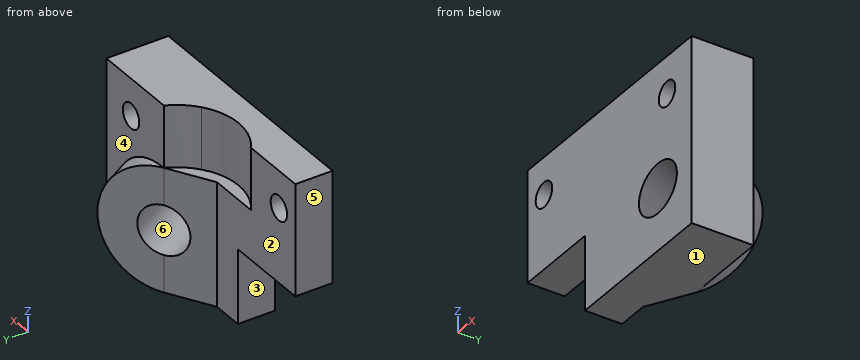
```python
from build123d import *

# Parameters (mm, degrees)
IZIM1_W                     = 35
IZIM1_H                     = 75
Y_KSEKLIK_EKSTR_ZYON1_DEPTH = 25
Y_KSEKLIK_EKSTR_ZYON2_DEPTH = 15
KES_EKSTR_ZYON1_DEPTH       = 25
Y_KSEKLIK_EKSTR_ZYON3_DEPTH = 25
IZIM3_R                     = 5
KES_EKSTR_ZYON2_DEPTH       = 25
IZIM4_R                     = 5
KES_EKSTR_ZYON3_DEPTH       = 26
Y_KSEKLIK_EKSTR_ZYON4_DEPTH = 50
Y_KSEKLIK_EKSTR_ZYON5_REACH = 41.151
IZIM7_R                     = 10
KES_EKSTR_ZYON4_DEPTH       = 40.150635095


with BuildPart() as part:
    # izim1 → Y_kseklik-Ekstr_zyon1 (new body)
    with BuildSketch(Plane(origin=(0, 0, 0), x_dir=(1, 0, 0), z_dir=(0, 1, 0))):
        with Locations((-17.5, 37.5)):
            Rectangle(IZIM1_W, IZIM1_H)
    extrude(amount=Y_KSEKLIK_EKSTR_ZYON1_DEPTH)

    # izim1_4 → Y_kseklik-Ekstr_zyon2 (add)
    with BuildSketch(Plane(origin=(0, 0, 0), x_dir=(1, 0, 0), z_dir=(0, 1, 0))):
        Polygon((-35, 75), (-65, 75), (-65, 45), (-100, 45), (-100, 0), (-35, 0), align=None)
    extrude(amount=Y_KSEKLIK_EKSTR_ZYON2_DEPTH)

    # izim2 → Kes-Ekstr_zyon1 (cut)
    with BuildSketch(Plane.XY):
        with BuildLine():
            Line((-42.912878475, 15), (-72.912878475, 15))
            ThreePointArc((-72.912878475, 15), (-57.912878475, 10), (-42.912878475, 15))
        make_face()
    extrude(amount=-KES_EKSTR_ZYON1_DEPTH, mode=Mode.SUBTRACT)

    # izim2_3 → Y_kseklik-Ekstr_zyon3 (add)
    with BuildSketch(Plane.XY):
        with BuildLine():
            ThreePointArc((-35, 25), (-38.30811914, 19.486992186), (-42.912878475, 15))
            Line((-42.912878475, 15), (-35, 15))
            Line((-35, 15), (-35, 25))
        make_face()
    extrude(amount=-Y_KSEKLIK_EKSTR_ZYON3_DEPTH)

    # izim3 → Kes-Ekstr_zyon2 (cut)
    with BuildSketch(Plane(origin=(0, 15, 0), x_dir=(1, 0, 0), z_dir=(0, 1, 0))):
        with Locations((-90, 15)):
            Circle(IZIM3_R)
    extrude(amount=-KES_EKSTR_ZYON2_DEPTH, mode=Mode.SUBTRACT)

    # izim4 → Kes-Ekstr_zyon3 (cut, through all)
    with BuildSketch(Plane(origin=(0, 25, 0), x_dir=(1, 0, 0), z_dir=(0, 1, 0))):
        with Locations((-15, 15)):
            Circle(IZIM4_R)
    extrude(amount=-KES_EKSTR_ZYON3_DEPTH, mode=Mode.SUBTRACT)

    # izim5 → Y_kseklik-Ekstr_zyon4 (add)
    with BuildSketch(Plane.XY.offset(-75)):
        Polygon((-35, 25), (-52.320508076, 15), (-35, 15), align=None)
    extrude(amount=Y_KSEKLIK_EKSTR_ZYON4_DEPTH)

    # Y_kseklik-Ekstr_zyon5: up to this face of the body (flat: up to its plane)
    y_kseklik_ekstr_zyon5_end = Plane(part.part.faces().sort_by_distance((-17.577106857, 25, -38.193961712))[0])
    # izim6 → Y_kseklik-Ekstr_zyon5 (add, up to the picked face)
    with BuildSketch(Plane(origin=(-19.575317547, 33.905444566, 0), x_dir=(0.866025404, 0.5, 0), z_dir=(-0.5, 0.866025404, 0)), mode=Mode.PRIVATE) as y_kseklik_ekstr_zyon5_sk1:
        with BuildLine():
            Line((-17.810889132, 25), (-17.810889132, 75))
            ThreePointArc((-17.810889132, 75), (7.189110868, 50), (-17.810889132, 25))
        make_face()
    y_kseklik_ekstr_zyon5_tool1 = split(extrude(y_kseklik_ekstr_zyon5_sk1.sketch, amount=-Y_KSEKLIK_EKSTR_ZYON5_REACH, mode=Mode.PRIVATE), bisect_by=y_kseklik_ekstr_zyon5_end, keep=Keep.BOTH, mode=Mode.PRIVATE)
    add(y_kseklik_ekstr_zyon5_tool1.solids().sort_by_distance((-25.811185, 30.305165, -50))[0])

    # izim7 → Kes-Ekstr_zyon4 (cut, through all)
    with BuildSketch(Plane(origin=(-19.575317547, 33.905444566, 0), x_dir=(0.866025404, 0.5, 0), z_dir=(-0.5, 0.866025404, 0))):
        with Locations((-17.810889132, 50)):
            Circle(IZIM7_R)
    extrude(amount=-KES_EKSTR_ZYON4_DEPTH, mode=Mode.SUBTRACT)


solid = part.part
```
The listing builds one solid part. Answer for the finished solid, in the listing's coordinates (mm). Face numbers are marked on the shaded views. A direction names the side the tool comes from. Give positions to 0.01 mm unless a question says otherwise; leave off trailing zeros. Order: outer loops, then holes, each group sorted by start corner. A loop starts at its lowest first (then second) coordinate and runs counter-clockwise, first axis right, second up. Notation, with made-up numbers: (44, 33.5) -> (94, 33.5) arc R24 cw to (94, 46.5) -> close; hole circle Ø6 at (71, -6). An arc over 180 degrees is marked (long way). Answer as CSV lines item,"result". Start each with the question number.
Q1. Which of the six approach directions +Z, -Z, +X, -X, +Y, -Y give full straight-line access (tool end or side, diameter ignored) to the marked faces 1, 2 and 3?
Q2. Determine the mould class of the marked faces 4, 5 and 6 for opening direction X: pulls with the +X half, pulls with the -X half, needs draft (parallel to the pull), parting line crosses it, or undercut.
Q3. A cutting plane is placed at C-C (z = -64.5). Determine the outline of the cut face in (x, y), then the cut area to 3 significant figures.
Q4. A cutting plane is placed at A-A (x = -90). Determine the outline of the cut face in (y, z), then the cut area to 3 significant figures.
Q5. Given pin 1 (8 mm diameter, centred on x = -15, z = -15, fed in from +Y); pin 2 (7.5 mm diameter, centred on x = -61.5, y = 16, fed in from +Z); pin 3 (8 mm diameter, centred on y = 28.5, z = -26.5, fed in from -X); pin 4 (17.5 mm diameter, centred on x = -25, z = -27, fed in from +Y), each flat-ended and moving along its own axis, determine where each tip first touches the part or whether it passes through.
Q6. A cutting plane is placed at D-D (x = -61). Determine the outline of the cut face in (y, z), then the cut area to 3 significant figures.
Q7. A cutting plane is placed at B-B (z = -15). Determine the outline of the cut face in (x, y).
Q8. Find the intervals of material crossed by L1, parallel to X at y = 7.75, z = -15; L2, parallel to Z at x = -90, y = 5.5; L3, parallel to Z at x = -15, y = 15.25, in increasing order.
Results found:
1,face 1,"-Z, +X, -X, +Y, -Y"
1,face 2,"+Z, -Z, -X, +Y"
1,face 3,"-Z, -X, +Y, -Y"
2,face 4,"needs draft"
2,face 5,"pulls with the -X half"
2,face 6,"undercut"
3,outline,"(-65, 0) -> (0, 0) -> (0, 25) -> (-11.48, 25) -> (-17.36, 35.18) -> (-52.32, 15) -> (-65, 15) -> close"
3,area,"1,530 mm2"
4,outline,"(0, -45) -> (15, -45) -> (15, -20) -> (0, -20) -> close; (0, -10) -> (15, -10) -> (15, 0) -> (0, 0) -> close"
4,area,"525 mm2"
5,pin 1,"through"
5,pin 2,"z = -25"
5,pin 3,"x = -35.87"
5,pin 4,"y = 34.29"
6,outline,"(0, -75) -> (15, -75) -> (15, -25) -> (10.19, -25) -> (10.19, 0) -> (0, 0) -> close"
6,area,"1,000 mm2"
7,outline,"(-100, 0) -> (-95, 0) -> (-95, 15) -> (-100, 15) -> close; (-85, 0) -> (-20, 0) -> (-20, 25) -> (-35, 25) arc R25 cw to (-72.91, 15) -> (-85, 15) -> close; (-10, 0) -> (0, 0) -> (0, 25) -> (-10, 25) -> close"
8,L1,"-100 to -95, -85 to -20, -10 to 0"
8,L2,"-45 to -20, -10 to 0"
8,L3,"-75 to -20, -10 to 0"
